```python
from build123d import *

# Parameters (mm, degrees)
SKETCH3_W                                            = 40
SKETCH3_H                                            = 25
BOSS_EXTRUDE2_DEPTH                                  = 5
CUT_EXTRUDE2_DEPTH                                   = 26.617376915
CUT_EXTRUDE2_DEPTH_BACK                              = 26.617376915
SKETCH4_R                                            = 7.5
SKETCH5_W                                            = 40
SKETCH5_H                                            = 10
BOSS_EXTRUDE3_DEPTH                                  = 20
CBORE_FOR_M3_HEXAGON_SOCKET_HEAD_CAP_SCR_D           = 3.4
CBORE_FOR_M3_HEXAGON_SOCKET_HEAD_CAP_SCR_CBORE_D     = 6.2
CBORE_FOR_M3_HEXAGON_SOCKET_HEAD_CAP_SCR_CBORE_DEPTH = 4
FILLET1_R                                            = 2
SKETCH9_W                                            = 22.5
SKETCH9_H                                            = 10
BOSS_EXTRUDE4_DEPTH                                  = 8
CHAMFER1_SIZE                                        = 5
M3_TAPPED_HOLE1_D                                    = 2.5
M3_TAPPED_HOLE1_DEPTH                                = 10
M3_TAPPED_HOLE1_TIP                                  = 0.751075774
FILLET2_R                                            = 3
M4_TAPPED_HOLE1_D                                    = 3.3
M4_TAPPED_HOLE1_DEPTH                                = 8
M4_TAPPED_HOLE1_TIP                                  = 0.991420021


with BuildPart() as part:
    # Sketch3 → Boss-Extrude2 (new, symmetric)
    with BuildSketch(Plane(origin=(0, 0, 0), x_dir=(1, 0, 0), z_dir=(0, 1, 0))):
        Rectangle(SKETCH3_W, SKETCH3_H)
    extrude(amount=BOSS_EXTRUDE2_DEPTH, both=True)

    # Sketch4 → Cut-Extrude2 (cut, two sides: drawn at the far end of the back side and taken through both)
    with BuildSketch(Plane(origin=(0, 5, 0), x_dir=(1, 0, 0), z_dir=(0, 1, 0)).offset(-CUT_EXTRUDE2_DEPTH_BACK)):
        with Locations(Location((0, 0, 0), (0, 0, 270))):
            Circle(SKETCH4_R)
    extrude(amount=CUT_EXTRUDE2_DEPTH + CUT_EXTRUDE2_DEPTH_BACK, mode=Mode.SUBTRACT)

    # Sketch5 → Boss-Extrude3 (add)
    with BuildSketch(Plane.XZ.offset(-5)):
        with Locations((0, 15)):
            Rectangle(SKETCH5_W, SKETCH5_H)
    extrude(amount=BOSS_EXTRUDE3_DEPTH)

    # CBORE for M3 Hexagon socket head cap screws1 (through all)
    with Locations(Plane(origin=(0, -5, 0), x_dir=(-1, 0, 0), z_dir=(0, -1, 0))):
        with Locations((0, 9.5), (8.227241336, -4.75), (-8.227241336, -4.75)):
            CounterBoreHole(CBORE_FOR_M3_HEXAGON_SOCKET_HEAD_CAP_SCR_D / 2, CBORE_FOR_M3_HEXAGON_SOCKET_HEAD_CAP_SCR_CBORE_D / 2, CBORE_FOR_M3_HEXAGON_SOCKET_HEAD_CAP_SCR_CBORE_DEPTH)

    # Fillet1
    fillet1_edges = [part.edges().sort_by_distance(p)[0] for p in [
        (5.197639771, -3, 5.406897522),
        (7.281330495, -3, 1.79783932),
        (-7.281330495, -3, 1.79783932),
        (-5.197639771, -3, 5.406897522),
        (2.083690725, -3, -7.204736842),
        (-2.083690725, -3, -7.204736842),
        (-0.781024968, -3, -12.5),
        (0.781024968, -3, -12.5),
    ]]
    fillet(fillet1_edges, radius=FILLET1_R)

    # Sketch9 → Boss-Extrude4 (add)
    with BuildSketch(Plane(origin=(20, 0, 0), x_dir=(0, 0, -1), z_dir=(1, 0, 0))):
        with Locations((1.25, -10)):
            Rectangle(SKETCH9_W, SKETCH9_H)
    boss_extrude4 = extrude(amount=-BOSS_EXTRUDE4_DEPTH)

    # Mirror1: Boss-Extrude4 across plane
    add(boss_extrude4.mirror(Plane(origin=(0, 0, 0), x_dir=(0, 0, 1), z_dir=(1, 0, 0))))

    # Chamfer1
    chamfer1_edges = [part.edges().sort_by_distance(p)[0] for p in [
        (16, -15, -12.5),
        (-16, -15, -12.5),
    ]]
    chamfer(chamfer1_edges, length=CHAMFER1_SIZE)

    # M3 Tapped Hole1
    with Locations(Plane(origin=(0, 5, 0), x_dir=(1, 0, 0), z_dir=(0, 1, 0))):
        with Locations((-16, 7.5), (-16, -15), (16, -15), (16, 7.5)):
            Hole(M3_TAPPED_HOLE1_D / 2, depth=M3_TAPPED_HOLE1_DEPTH)
            with Locations((0, 0, -(M3_TAPPED_HOLE1_DEPTH + M3_TAPPED_HOLE1_TIP / 2))):  # 118° drill point
                Cone(0, M3_TAPPED_HOLE1_D / 2, M3_TAPPED_HOLE1_TIP, mode=Mode.SUBTRACT)

    # Fillet2
    fillet2_edges = [part.edges().sort_by_distance(p)[0] for p in [
        (12, -10, 10),
        (-12, -10, 10),
    ]]
    fillet(fillet2_edges, radius=FILLET2_R)

    # M4 Tapped Hole1
    with Locations(Plane.XY.offset(20)):
        with Locations((0, -5)):
            Hole(M4_TAPPED_HOLE1_D / 2, depth=M4_TAPPED_HOLE1_DEPTH)
            with Locations((0, 0, -(M4_TAPPED_HOLE1_DEPTH + M4_TAPPED_HOLE1_TIP / 2))):  # 118° drill point
                Cone(0, M4_TAPPED_HOLE1_D / 2, M4_TAPPED_HOLE1_TIP, mode=Mode.SUBTRACT)


solid = part.part
```
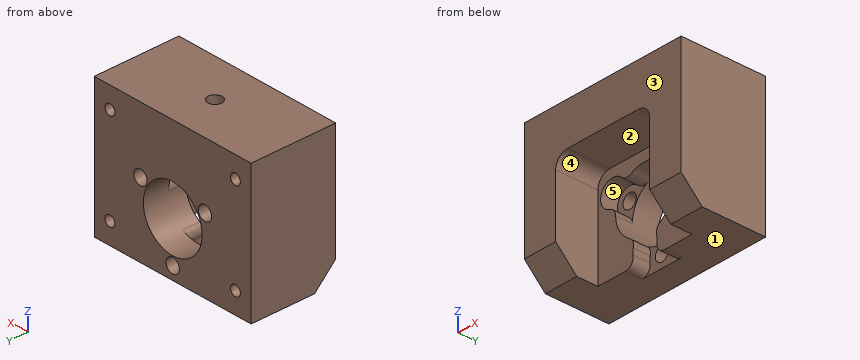
Check sheet for the modelled part. Datum: model origin and axes. Units: mm. Face numbers are marked on the shaded views. A direction names the side the tool comes from. Round coordinates to 2 decimals unless told otherwise and drop trailing zeros. Order: outer loops, then holes, each group sorted by start corner. A loop starts at its lowest first (then second) coordinate and runs counter-clockwise, first axis right, second up. Notation, with made-up numbers: (58.5, -36) -> (72.5, -36) arc R33 ccw to (72.5, -1) -> close; hole circle Ø6 at (-8.5, -32.75). An arc over 180 degrees is marked (long way). One line per item, written item: value. Start each with the question number.
Q1. Mould release check, pull along Z, two halves, no side actions. Record for the marked faces 3, 4 and 5: pulls with the +Z half, pulls with the -Z half, needs draft (parallel to the pull), parting line crosses it, or undercut.
Q2. Cross-section at D-D (y = -11). Record the boundary of the cut face in (x, z).
Q3. Cross-section at A-A (y = -0.5). Give the number of separate pieces and of enclosed holes in the cut face, and give its area (3 significant figures).
Q4. Thickness scan on line 1 (X direction, y = -1.75, z = 0); line 2 (X direction, y = 2.25, z = -8); line 3 (X direction, y = -11.25, z = 5). Record the ranges inside material, lowest first.
Q5. Set-up check for the marked faces 1 and 2: record each of +Z, -Z, +X, -X, +Y, -Y from which the full face is reachable in a straight line by a thin tool's end or side.
Q6. Gauge pin test, flat ends, axial feed: pin 1 Ø11.5 at (x, z) = (1, 3.5) entering from -Y; pin 2 Ø3 at (x, z) = (16, -7.5) entering from +Y; pin 3 Ø1.5 at (x, z) = (-5, 3.5) entering from +Y; pin 4 Ø8 at (x, y) = (-6.5, -12) entering from -Z. Record the tip position at first contact, or that the pin passes through.
Q7. Cross-section at C-C (z = 4.75). Record the boundary of the cut face in (x, y).
Q8. Cross-section at B-B (x = -7). Record the boundary of the cut face in (y, z).
Completed:
1. face 3: needs draft
1. face 4: pulls with the -Z half
1. face 5: undercut
2. outline: (-20, -11.5) -> (-12, -11.5) -> (-12, 7) arc R3 cw to (-9, 10) -> (9, 10) arc R3 cw to (12, 7) -> (12, -11.5) -> (20, -11.5) -> (20, 20) -> (-20, 20) -> close
3. separate pieces: 1
3. enclosed holes: 8
3. area: 1,080 mm²
4. line 1: x = -20 to -7.51, 7.51 to 20
4. line 2: x = -20 to -17.15, -14.85 to -0.8, 0.8 to 14.85, 17.15 to 20
4. line 3: x = -20 to -12, 12 to 20
5. face 1: -Z, +X, -X, +Y, -Y
5. face 2: -Z, -Y
6. pin 1: stops at y = -5
6. pin 2: stops at y = 5
6. pin 3: passes through
6. pin 4: stops at z = 9.6
7. outline: (-20, -15) -> (-12, -15) -> (-12, -5) -> (-11.33, -5) -> (-11.33, -1) -> (-9.93, -1) -> (-9.93, 5) -> (-20, 5) -> close; (-6.53, -1) -> (-5.8, -1) -> (-5.8, 5) -> (-6.53, 5) -> close; (5.8, -1) -> (6.53, -1) -> (6.53, 5) -> (5.8, 5) -> close; (9.93, -1) -> (11.33, -1) -> (11.33, -5) -> (12, -5) -> (12, -15) -> (20, -15) -> (20, 5) -> (9.93, 5) -> close
8. outline: (-15, 10) -> (-5, 10) -> (-5, 7.6) -> (-1, 7.6) -> (-1, 5.93) -> (5, 5.93) -> (5, 20) -> (-15, 20) -> close; (-5, -12.5) -> (5, -12.5) -> (5, -2.69) -> (-5, -2.69) -> close; (-1, 2.69) -> (5, 2.69) -> (5, 3.57) -> (-1, 3.57) -> close
